```python
from build123d import *

# Parameters (mm, degrees)
LINEAR_AUSTRAGEN1_DEPTH         = 34
SCHNITT_LINEAR_AUSTRAGEN1_REACH = 79.498
SKIZZE8_W                       = 42
SKIZZE8_H                       = 24


with BuildPart() as part:
    # Skizze1 → Linear austragen1 (new body)
    with BuildSketch(Plane.XY):
        with BuildLine():
            Line((-22, -1), (-22, -12.5))
            Line((-22, -12.5), (65, -12.5))
            Line((65, -12.5), (65, 12.5))
            Line((65, 12.5), (-22, 12.5))
            Line((-22, 12.5), (-22, 1))
            Line((-22, 1), (-7.433034374, 1))
            ThreePointArc((-7.433034374, 1), (0, 7.5), (7.433034374, 1))
            Line((7.433034374, 1), (11.5, 1))
            Line((11.5, 1), (11.5, -1))
            Line((11.5, -1), (7.433034374, -1))
            ThreePointArc((7.433034374, -1), (0, -7.5), (-7.433034374, -1))
            Line((-7.433034374, -1), (-22, -1))
        make_face()
    extrude(amount=-LINEAR_AUSTRAGEN1_DEPTH)

    # Skizze8 → Schnitt-Linear austragen1 (cut, up to next)
    with BuildSketch(Plane.XZ.offset(12.5), mode=Mode.PRIVATE) as schnitt_linear_austragen1_sk1:
        with Locations((44, -12)):
            Rectangle(SKIZZE8_W, SKIZZE8_H)
    schnitt_linear_austragen1_tool1 = extrude(schnitt_linear_austragen1_sk1.sketch, amount=-SCHNITT_LINEAR_AUSTRAGEN1_REACH, mode=Mode.PRIVATE) & part.part
    add(schnitt_linear_austragen1_tool1.solids().sort_by_distance((44, -12.5, -12))[0], mode=Mode.SUBTRACT)


solid = part.part
```
Design review of the part built by this model. Coordinates are the model's own, in mm. A direction names the side the tool comes from. Coordinates: 2 decimals unless noted, no trailing zeros. Loops run counter-clockwise (first coordinate to the right, second up) from the corner with the lowest first, then second, coordinate; pieces in that order, holes last.
Q1. We need section B-B on x = 2. State the section outline as (y, z) points, and give its area (3 significant figures).
Reported:
outline: (-12.5, -34) - (-7.23, -34) - (-7.23, 0) - (-12.5, 0) - close; (7.23, -34) - (12.5, -34) - (12.5, 0) - (7.23, 0) - close
area: 358 mm2
Q2. We need section A-A on y = -3.5. State the section outline as (x, z) points.
Reported:
outline: (-22, -34) - (-6.63, -34) - (-6.63, 0) - (-22, 0) - close; (6.63, -34) - (65, -34) - (65, -24) - (23, -24) - (23, 0) - (6.63, 0) - close
Q3. We need section C-C on z = -29. State the section outline as (x, y) points, and give its area (3 significant figures).
Reported:
outline: (-22, -12.5) - (65, -12.5) - (65, 12.5) - (-22, 12.5) - (-22, 1) - (-7.43, 1) arc R7.5 cw to (7.43, 1) - (11.5, 1) - (11.5, -1) - (7.43, -1) arc R7.5 cw to (-7.43, -1) - (-22, -1) - close
area: 1,960 mm2
Q4. Tool access review of faces 4 (the face through (11, -12.5, -21)), 5 (the face through (-0.15, 7.5, -16.76)), 6 (the face through (5, 6, 0)), 7 (the face through (-15, 1, -17)), 8 (the face through (23, 0, -12)): name each direction out of +Z, -Z, +X, -X, +Y, -Y from which nothing blocks a thin tool from reaching the whole face with its end or side.
Reported:
face 4: +Z, -Z, +X, -X, -Y
face 5: +Z, -Z
face 6: +Z, +X, -X, +Y, -Y
face 7: +Z, -Z, -X
face 8: +Z, +X, +Y, -Y
Q5. For pin 1 (1 mm diameter, centred on y = 0, z = -21.5, fed in from -X); pin 2 (3 mm diameter, centred on x = 44.5, y = 5, fed in from +Z); pin 3 (5 mm diameter, centred on y = -7.5, z = -13, fed in from +X), all flat-tipped, find the tip position at first contact; note any pin that passes through.
Reported:
pin 1: stops at x = 11.5
pin 2: stops at z = -24
pin 3: stops at x = 23
Q6. To check wall thickness, follow line 1 (Y direction, x = -9, z = -15); line 2 (X direction, y = -9.25, z = -3.5); line 3 (Z direction, x = 42, y = -2). State the ranges of each line that lie inside material, in increasing order.
Reported:
line 1: y = -12.5 to -1, 1 to 12.5
line 2: x = -22 to 23
line 3: z = -34 to -24
Q7. We need section D-D on y = 10.5. State the section outline as (x, z) points.
Reported:
outline: (-22, -34) - (65, -34) - (65, -24) - (23, -24) - (23, 0) - (-22, 0) - close
Q8. The part is to be moulded in two halves that separate along X. For faces 1 (the face through (11.5, 0, -17)), 2 (the face through (0.15, -7.5, -16.76)), 3 (the face through (9, -1, -17)), say which applies: +X half, -X half, draft (parallel to the pull), parting line (faces both ways), or undercut.
Reported:
face 1: -X half
face 2: undercut
face 3: draft
